Part model, mm, in its own coordinate system. A direction names the side the tool comes from. Round coordinates to 2 decimals unless told otherwise and drop trailing zeros. Loops run counter-clockwise (first coordinate to the right, second up) from the corner with the lowest first, then second, coordinate; pieces in that order, holes last. Notation, with made-up numbers: (57.25, 86) -> (68.25, 86) arc R14 cw to (68.25, 90) -> close; hole circle Ø5 at (84.25, -28.75). An arc over 180 degrees is marked (long way). Use a Markdown table: item, result. Add a question column.
Item 1: Flat gauge pins, fed straight in: pin 1 (1.6 mm diameter, centred on x = -72, z = 1, fed in from -Y); pin 2 (1 mm diameter, centred on x = -71, z = 1, fed in from +Y); pin 3 (1 mm diameter, centred on y = 59, z = 1, fed in from -X); pin 4 (1.8 mm diameter, centred on x = 63.5, y = -60.325, fed in from +Z). Where does each tip first touch, or does it go through?
Item 2: Cut at C-C, the plane y = 0. List the corners of the cut face in (x, z) (3 decimals).
Item 3: Probe line 1 (X direction, y = 8, z = 1.4) (3 decimals); line 2 (X direction, y = -7.5, z = 2.05) (3 decimals); line 3 (Y direction, x = 0.5, z = 1.45). List the from-to ranges inside material, lowest first. Write a range as [from, to].
Item 4: Two-plate mould, pull along Y, no slides. Class faces 1 (the face through (-68.154, 32.474, 1.61)), 2 (the face through (6, 5, 0)), 3 (the face through (-35.945, 41.75, 1.565)): pulls with the +Y half, pulls with the -Y half, needs draft (parallel to the pull), parting line crosses it, or undercut.
Item 5: Cut at A-A, the plane x = 0. List the corners of the cut face in (y, z) (3 decimals).
Item 6: Cut at D-D, the plane x = 25. List the corners of the cut face in (y, z) (3 decimals), plus the area to 3 significant figures.
Item 7: Cut at B-B, the plane y = -21.5. List the corners of the cut face in (x, z) (3 decimals).
Item 8: Which spindle directions (+Z, -Z, +X, -X, +Y, -Y) get a long thin tool onto all of the face, cutting with end or side? Do faces 4 (the face through (-62.904, 38.738, 1.565)), 5 (the face through (62.4, 61.5, 1.3)), 6 (the face through (-71, 57.15, 2)), 7 (the face through (35.945, 41.75, 1.565)). Say none if no direction does.
```python
from build123d import *

# Parameters (mm, degrees)
BOSS_EXTRUDE1_DEPTH           = 3.175
MIRROR2_COPY_1_DEPTH          = 3.175
INTERNAL_SHARPS_R             = 9.525
IMU_MOUNTING_DEPTH            = 3.175
IMU_MOUNTING_HOLES_AT_2_COUNT = 2
IMU_MOUNTING_HOLES_AT_2_PITCH = 21.59
FILLET4_R                     = 6.35
SKETCH6_R                     = 6.35
MATERIAL_REMOVAL_DEPTH        = 99.935771608


with BuildPart() as part:
    # Sketch1 → Boss-Extrude1 (new body)
    with BuildSketch(Plane.XY):
        with BuildLine():
            Line((9.434743879, 15.24), (0, 15.24))
            Line((0, 15.24), (0, 0))
            Line((0, 0), (12.7, 0))
            Line((12.7, 0), (12.7, 12.892596045))
            Line((12.7, 12.892596045), (51.712045103, 51.904641149))
            ThreePointArc((51.712045103, 51.904641149), (62.784313673, 54.107052302), (69.05625, 44.720436252))
            Line((69.05625, 44.720436252), (69.05625, 0))
            Line((69.05625, 0), (73.025, 0))
            Line((73.025, 0), (73.025, 57.15))
            Line((73.025, 57.15), (69.85, 57.15))
            Line((69.85, 57.15), (69.85, 60.325))
            ThreePointArc((69.85, 60.325), (65.930039796, 66.191635031), (59.009871939, 64.815128061))
            Line((59.009871939, 64.815128061), (9.434743879, 15.24))
        make_face()
    boss_extrude1 = extrude(amount=BOSS_EXTRUDE1_DEPTH)

    # Sketch11 → CSK for #4 Flat Head Machine Screw1 (revolve, cut)
    with BuildSketch(Plane(origin=(63.5, 60.325, 3.175), x_dir=(0, -1, 0), z_dir=(1, 0, 0))):
        Polygon((0, 0), (0, 3.175), (1.4732, 3.175), (1.4732, 2.030745349), (3.2385, 0), align=None)
    csk_for_4_flat_head_machine_screw1 = revolve(axis=Axis((63.5, 60.325, 9.525), (0, 0, -1)), mode=Mode.SUBTRACT)

    # Mirror1: Boss-Extrude1, CSK for #4 Flat Head Machine Screw1 across plane
    add(boss_extrude1.mirror(Plane.ZX))
    add(csk_for_4_flat_head_machine_screw1.mirror(Plane.ZX), mode=Mode.SUBTRACT)

    # Mirror2: Boss-Extrude1, CSK for #4 Flat Head Machine Screw1 across plane
    add(boss_extrude1.mirror(Plane(origin=(0, 0, 0), x_dir=(0, 0, 1), z_dir=(1, 0, 0))))
    add(csk_for_4_flat_head_machine_screw1.mirror(Plane(origin=(0, 0, 0), x_dir=(0, 0, 1), z_dir=(1, 0, 0))), mode=Mode.SUBTRACT)

    # Mirror2 copy 1 sketch → Mirror2 copy 1 (add)
    with BuildSketch(Plane(origin=(0, 0, 0), x_dir=(-1, 0, 0), z_dir=(0, 0, 1))):
        with BuildLine():
            Line((9.434743879, 15.24), (0, 15.24))
            Line((0, 15.24), (0, 0))
            Line((0, 0), (12.7, 0))
            Line((12.7, 0), (12.7, 12.892596045))
            Line((12.7, 12.892596045), (51.712045103, 51.904641149))
            ThreePointArc((51.712045103, 51.904641149), (62.784313673, 54.107052302), (69.05625, 44.720436252))
            Line((69.05625, 44.720436252), (69.05625, 0))
            Line((69.05625, 0), (73.025, 0))
            Line((73.025, 0), (73.025, 57.15))
            Line((73.025, 57.15), (69.85, 57.15))
            Line((69.85, 57.15), (69.85, 60.325))
            ThreePointArc((69.85, 60.325), (65.930039796, 66.191635031), (59.009871939, 64.815128061))
            Line((59.009871939, 64.815128061), (9.434743879, 15.24))
        make_face()
    extrude(amount=MIRROR2_COPY_1_DEPTH)

    # Mirror2 copy 2 sketch → Mirror2 copy 2 (revolve, cut)
    with BuildSketch(Plane(origin=(-63.5, -60.325, 3.175), x_dir=(0, 1, 0), z_dir=(-1, 0, 0))):
        Polygon((0, 0), (0, 3.175), (1.4732, 3.175), (1.4732, 2.030745349), (3.2385, 0), align=None)
    revolve(axis=Axis((-63.5, -60.325, 9.525), (0, 0, -1)), mode=Mode.SUBTRACT)

    # INTERNAL-SHARPS
    internal_sharps_edges = [part.edges().sort_by_distance(p)[0] for p in [
        (-9.434743879, 15.24, 1.5875),
        (-12.7, 12.892596045, 1.5875),
        (9.434743879, 15.24, 1.5875),
        (12.7, 12.892596045, 1.5875),
        (9.434743879, -15.24, 1.5875),
        (12.7, -12.892596045, 1.5875),
        (-12.7, -12.892596045, 1.5875),
        (-9.434743879, -15.24, 1.5875),
    ]]
    fillet(internal_sharps_edges, radius=INTERNAL_SHARPS_R)

    # Sketch13 → IMU-MOUNTING (add)
    with BuildSketch(Plane.XY):
        with BuildLine():
            Line((-73.025, 44.45), (-73.025, 12.7))
            Line((-73.025, 12.7), (-67.945, 12.7))
            ThreePointArc((-67.945, 12.7), (-62.895851895, 18.339020045), (-69.05625, 22.736967161))
            Line((-69.05625, 22.736967161), (-69.05625, 34.413032839))
            ThreePointArc((-69.05625, 34.413032839), (-62.895851895, 38.810979955), (-67.945, 44.45))
            Line((-67.945, 44.45), (-73.025, 44.45))
        make_face()
    extrude(amount=IMU_MOUNTING_DEPTH)

    # Sketch15 → IMU-MOUNTING-HOLES (revolve, cut)
    with BuildSketch(Plane(origin=(-67.945, 17.78, 3.175), x_dir=(0, -1, 0), z_dir=(1, 0, 0))):
        Polygon((0, 0), (0, 3.175), (1.4732, 3.175), (1.4732, 2.030745349), (3.2385, 0), align=None)
    imu_mounting_holes = revolve(axis=Axis((-67.945, 17.78, 9.525), (0, 0, -1)), mode=Mode.SUBTRACT)

    # IMU-MOUNTING-HOLES at 2: IMU-MOUNTING-HOLES ×2
    with Locations(*[(0, i * IMU_MOUNTING_HOLES_AT_2_PITCH, 0) for i in range(1, IMU_MOUNTING_HOLES_AT_2_COUNT)]):
        add(imu_mounting_holes, mode=Mode.SUBTRACT)

    # Fillet4
    fillet4_edges = [part.edges().sort_by_distance(p)[0] for p in [
        (-69.05625, 44.45, 1.5875),
        (-69.05625, 12.7, 1.5875),
        (-69.05625, 22.736967161, 1.5875),
        (-69.05625, 34.413032839, 1.5875),
    ]]
    fillet(fillet4_edges, radius=FILLET4_R)

    # Sketch6 → MATERIAL-REMOVAL (cut, through all)
    with BuildSketch(Plane(origin=(0, 0, 0), x_dir=(-1, 0, 0), z_dir=(0, 0, -1))):
        Circle(SKETCH6_R)
    extrude(amount=-MATERIAL_REMOVAL_DEPTH, mode=Mode.SUBTRACT)


solid = part.part
```
A:
| question | item | result |
|---|---|---|
| 1 | pin 1 | stops at y = -57.15 |
| 1 | pin 2 | stops at y = 57.15 |
| 1 | pin 3 | stops at x = -69.85 |
| 1 | pin 4 | passes through |
| 2 | outline | (-73.025, 0) -> (-69.056, 0) -> (-69.056, 3.175) -> (-73.025, 3.175) -> close; (-12.7, 0) -> (-6.35, 0) -> (-6.35, 3.175) -> (-12.7, 3.175) -> close; (6.35, 0) -> (12.7, 0) -> (12.7, 3.175) -> (6.35, 3.175) -> close; (69.056, 0) -> (73.025, 0) -> (73.025, 3.175) -> (69.056, 3.175) -> close |
| 3 | line 1 | x = [-73.025, -69.045], [-12.7, 12.7], [69.056, 73.025] |
| 3 | line 2 | x = [-73.025, -69.056], [-12.7, 12.7], [69.056, 73.025] |
| 3 | line 3 | y = [-15.24, -6.33], [6.33, 15.24] |
| 4 | face 1 | undercut |
| 4 | face 2 | needs draft |
| 4 | face 3 | pulls with the +Y half |
| 5 | outline | (-15.24, 0) -> (-6.35, 0) -> (-6.35, 3.175) -> (-15.24, 3.175) -> close; (6.35, 0) -> (15.24, 0) -> (15.24, 3.175) -> (6.35, 3.175) -> close |
| 6 | outline | (-30.805, 0) -> (-25.193, 0) -> (-25.193, 3.175) -> (-30.805, 3.175) -> close; (25.193, 0) -> (30.805, 0) -> (30.805, 3.175) -> (25.193, 3.175) -> close |
| 6 | area | 35.6 mm^2 |
| 7 | outline | (-73.025, 0) -> (-69.056, 0) -> (-69.056, 3.175) -> (-73.025, 3.175) -> close; (-21.307, 0) -> (-15.695, 0) -> (-15.695, 3.175) -> (-21.307, 3.175) -> close; (15.695, 0) -> (21.307, 0) -> (21.307, 3.175) -> (15.695, 3.175) -> close; (69.056, 0) -> (73.025, 0) -> (73.025, 3.175) -> (69.056, 3.175) -> close |
| 8 | face 4 | +Z, -Z |
| 8 | face 5 | +Z |
| 8 | face 6 | +Z, -Z, -X, +Y |
| 8 | face 7 | +Z, -Z, +Y |
